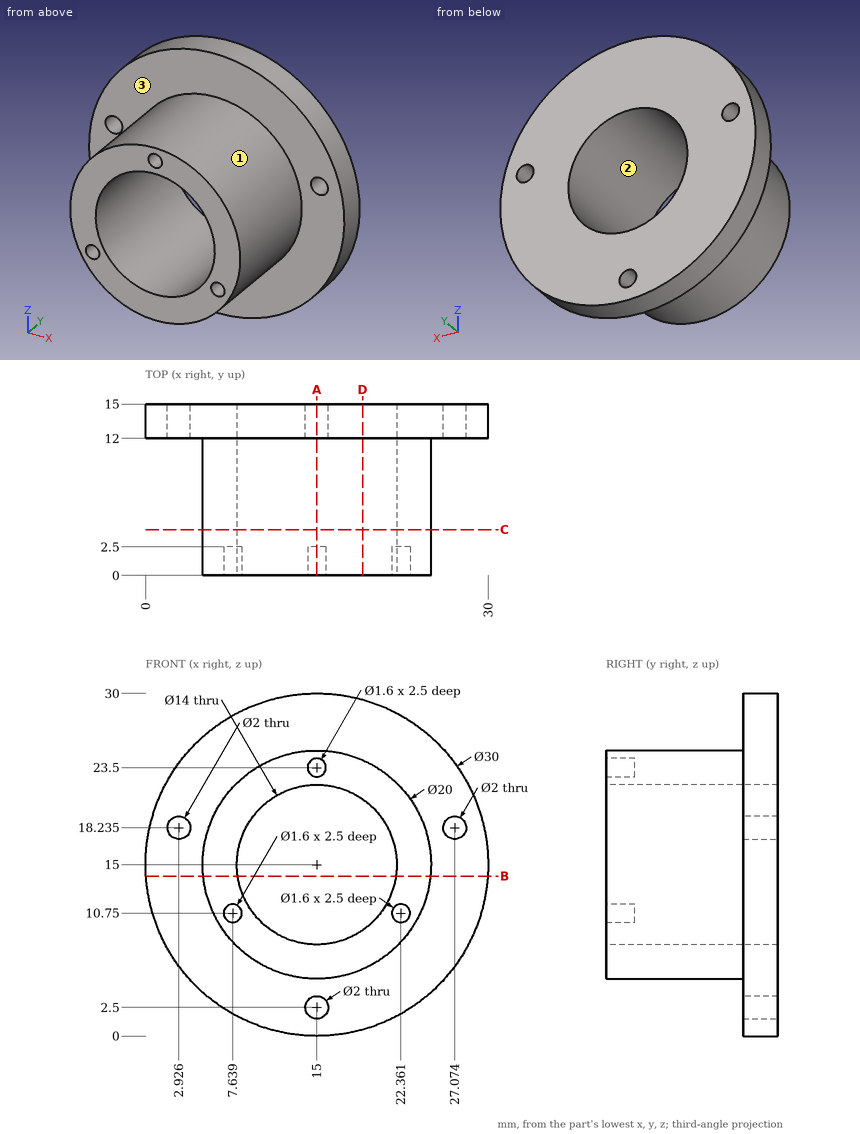
Part print with two shaded views. Sizes in mm from the minimum x, y, z corner. Give positions to 0.01 mm unless a question says otherwise; leave off trailing zeros. Order: outer loops, then holes, each group sorted by start corner. A loop starts at its lowest first (then second) coordinate and runs counter-clockwise, first axis right, second up.
(1) Drill centre lines: L1, parallel to X at y = 7.5, z = 15; L2, parallel to X at y = 1.1, z = 10.75; L3, parallel to Y at x = 13, z = 25. Where is each one in solid material? Low to high.
(2) Mould opens along Z. For the marked faces 1, 2 and 3 say: released by +Z, released by -Z, zero draft, split by the parting line, or undercut.
(3) Saw through at C-C, the plane y = 4. Give the cut face in (x, z).
(4) Flat gauge pins, fed straight in: pin 1 (2 mm diameter, centred on x = 13, y = 9, fed in from +Z); pin 2 (1.4 mm diameter, centred on x = 7.64, z = 10.75, fed in from -Y); pin 3 (5 mm diameter, centred on y = 11.5, z = 12, fed in from +X). Where does each tip first touch, or does it go through?
(5) Saw through at A-A, the plane x = 15. Give the cut face in (y, z).
(6) Saw through at D-D, the plane x = 19. Give the cut face in (y, z) (1 decimal).
(7) Saw through at B-B, the plane z = 14. Give the cut face in (x, y).
Results found:
1. L1: x = 5 to 8, 22 to 25
1. L2: x = 5.95 to 6.84, 8.44 to 9.44, 20.56 to 21.56, 23.16 to 24.05
1. L3: y = 12 to 15
2. face 1: split by the parting line
2. face 2: undercut
2. face 3: zero draft
3. outline: circle Ø20 at (15, 15); hole circle Ø14 at (15, 15)
4. pin 1: stops at z = 24.95
4. pin 2: stops at y = 2.5
4. pin 3: stops at x = 29.99
5. outline: (0, 5) - (12, 5) - (12, 3.5) - (15, 3.5) - (15, 8) - (0, 8) - close; (0, 22) - (15, 22) - (15, 30) - (12, 30) - (12, 25) - (0, 25) - (0, 24.3) - (2.5, 24.3) - (2.5, 22.7) - (0, 22.7) - close; (12, 0) - (15, 0) - (15, 1.5) - (12, 1.5) - close
6. outline: (0, 5.8) - (12, 5.8) - (12, 0.5) - (15, 0.5) - (15, 9.3) - (0, 9.3) - close; (0, 20.7) - (15, 20.7) - (15, 29.5) - (12, 29.5) - (12, 24.2) - (0, 24.2) - close
7. outline: (0.03, 12) - (5.05, 12) - (5.05, 0) - (8.07, 0) - (8.07, 15) - (0.03, 15) - close; (21.93, 0) - (24.95, 0) - (24.95, 12) - (29.97, 12) - (29.97, 15) - (21.93, 15) - close
